from build123d import *

# Parameters (mm, degrees)
SKETCH1_W           = 50.8
SKETCH1_H           = 50.8
SKETCH1_W_2         = 44.45
BOSS_EXTRUDE1_DEPTH = 6.35
FILLET2_R           = 3.175
SKETCH2_R           = 6.35
BOSS_EXTRUDE3_DEPTH = 6.35
BOSS_EXTRUDE4_START = -6.35
SKETCH4_R           = 6.35
BOSS_EXTRUDE4_DEPTH = 6.35
CUT_EXTRUDE1_REACH  = 164.453
SKETCH2_4_R         = 4.49961
SKETCH2_4_R_2       = 1.9939
BOSS_EXTRUDE5_DEPTH = 127


with BuildPart() as part:
    # Sketch1 → Boss-Extrude1 (new body)
    with BuildSketch(Plane(origin=(0, 0, 0), x_dir=(1, 0, 0), z_dir=(0, 1, 0))):
        Polygon((-146.05, 25.4), (-127, 25.4), (-127, -25.4), (-146.05, -25.4), (-146.05, -31.75), (146.05, -31.75), (146.05, -25.4), (127, -25.4), (127, 25.4), (146.05, 25.4), (146.05, 31.75), (-146.05, 31.75), align=None)
        with Locations((-31.75, 0)):
            Rectangle(SKETCH1_W, SKETCH1_H, mode=Mode.SUBTRACT)
        with Locations((-92.075, 0)):
            Rectangle(SKETCH1_W_2, SKETCH1_H, mode=Mode.SUBTRACT)
        with Locations((31.75, 0)):
            Rectangle(SKETCH1_W, SKETCH1_H, mode=Mode.SUBTRACT)
        with Locations((92.075, 0)):
            Rectangle(SKETCH1_W_2, SKETCH1_H, mode=Mode.SUBTRACT)
    extrude(amount=-BOSS_EXTRUDE1_DEPTH)

    # Fillet2
    fillet2_edges = [part.edges().sort_by_distance(p)[0] for p in [
        (-146.05, -6.35, 28.575),
        (-146.05, 0, 28.575),
        (-146.05, -6.35, -28.575),
        (-146.05, 0, -28.575),
        (146.05, -6.35, -28.575),
        (146.05, 0, -28.575),
        (146.05, -6.35, 28.575),
        (146.05, 0, 28.575),
    ]]
    fillet(fillet2_edges, radius=FILLET2_R - 0.0001)  # a hair under: the kernel refuses the full size

    # Sketch2 → Boss-Extrude3 (add)
    with BuildSketch(Plane.XY.offset(31.75)):
        with Locations((-142.875, -3.175)):
            Circle(SKETCH2_R)
    extrude(amount=-BOSS_EXTRUDE3_DEPTH)

    # Sketch4 → Boss-Extrude4 (add)
    with BuildSketch(Plane(origin=(0, 0, -31.75), x_dir=(-1, 0, 0), z_dir=(0, 0, -1)).offset(BOSS_EXTRUDE4_START)):
        with Locations((142.875, -3.175)):
            Circle(SKETCH4_R)
    extrude(amount=BOSS_EXTRUDE4_DEPTH)

    # Cut-Extrude1: up to this face of the body (flat: up to its plane)
    cut_extrude1_end = Plane(part.part.faces().sort_by_distance((-5.43222234, -3.175, -31.75))[0])
    # Sketch2<4> → Cut-Extrude1 (cut, up to the picked face)
    with BuildSketch(Plane.XY.offset(31.75), mode=Mode.PRIVATE) as cut_extrude1_sk1:
        with Locations((-142.875, -3.175)):
            Circle(SKETCH2_4_R)
    cut_extrude1_tool1 = split(extrude(cut_extrude1_sk1.sketch, amount=-CUT_EXTRUDE1_REACH, mode=Mode.PRIVATE), bisect_by=cut_extrude1_end, keep=Keep.BOTH, mode=Mode.PRIVATE)
    # Sketch2<4> → Cut-Extrude1 (cut, up to the picked face)
    with BuildSketch(Plane.XY.offset(31.75), mode=Mode.PRIVATE) as cut_extrude1_sk2:
        with Locations((-92.075, -3.175)):
            Circle(SKETCH2_4_R_2)
    cut_extrude1_tool2 = split(extrude(cut_extrude1_sk2.sketch, amount=-CUT_EXTRUDE1_REACH, mode=Mode.PRIVATE), bisect_by=cut_extrude1_end, keep=Keep.BOTH, mode=Mode.PRIVATE)
    # Sketch2<4> → Cut-Extrude1 (cut, up to the picked face)
    with BuildSketch(Plane.XY.offset(31.75), mode=Mode.PRIVATE) as cut_extrude1_sk3:
        with Locations((-31.75, -3.175)):
            Circle(SKETCH2_4_R_2)
    cut_extrude1_tool3 = split(extrude(cut_extrude1_sk3.sketch, amount=-CUT_EXTRUDE1_REACH, mode=Mode.PRIVATE), bisect_by=cut_extrude1_end, keep=Keep.BOTH, mode=Mode.PRIVATE)
    # Sketch2<4> → Cut-Extrude1 (cut, up to the picked face)
    with BuildSketch(Plane.XY.offset(31.75), mode=Mode.PRIVATE) as cut_extrude1_sk4:
        with Locations((31.75, -3.175)):
            Circle(SKETCH2_4_R_2)
    cut_extrude1_tool4 = split(extrude(cut_extrude1_sk4.sketch, amount=-CUT_EXTRUDE1_REACH, mode=Mode.PRIVATE), bisect_by=cut_extrude1_end, keep=Keep.BOTH, mode=Mode.PRIVATE)
    # Sketch2<4> → Cut-Extrude1 (cut, up to the picked face)
    with BuildSketch(Plane.XY.offset(31.75), mode=Mode.PRIVATE) as cut_extrude1_sk5:
        with Locations((92.075, -3.175)):
            Circle(SKETCH2_4_R_2)
    cut_extrude1_tool5 = split(extrude(cut_extrude1_sk5.sketch, amount=-CUT_EXTRUDE1_REACH, mode=Mode.PRIVATE), bisect_by=cut_extrude1_end, keep=Keep.BOTH, mode=Mode.PRIVATE)
    # Sketch2<4> → Cut-Extrude1 (cut, up to the picked face)
    with BuildSketch(Plane.XY.offset(31.75), mode=Mode.PRIVATE) as cut_extrude1_sk6:
        with Locations((-120.65, -3.175)):
            Circle(SKETCH2_4_R_2)
    cut_extrude1_tool6 = split(extrude(cut_extrude1_sk6.sketch, amount=-CUT_EXTRUDE1_REACH, mode=Mode.PRIVATE), bisect_by=cut_extrude1_end, keep=Keep.BOTH, mode=Mode.PRIVATE)
    # Sketch2<4> → Cut-Extrude1 (cut, up to the picked face)
    with BuildSketch(Plane.XY.offset(31.75), mode=Mode.PRIVATE) as cut_extrude1_sk7:
        with Locations((61.9125, -3.175)):
            Circle(SKETCH2_4_R_2)
    cut_extrude1_tool7 = split(extrude(cut_extrude1_sk7.sketch, amount=-CUT_EXTRUDE1_REACH, mode=Mode.PRIVATE), bisect_by=cut_extrude1_end, keep=Keep.BOTH, mode=Mode.PRIVATE)
    # Sketch2<4> → Cut-Extrude1 (cut, up to the picked face)
    with BuildSketch(Plane.XY.offset(31.75), mode=Mode.PRIVATE) as cut_extrude1_sk8:
        with BuildLine():
            Line((135.255, -1.1811), (142.875, -1.1811))
            ThreePointArc((142.875, -1.1811), (144.8689, -3.175), (142.875, -5.1689))
            Line((142.875, -5.1689), (135.255, -5.1689))
            ThreePointArc((135.255, -5.1689), (133.2611, -3.175), (135.255, -1.1811))
        make_face()
    cut_extrude1_tool8 = split(extrude(cut_extrude1_sk8.sketch, amount=-CUT_EXTRUDE1_REACH, mode=Mode.PRIVATE), bisect_by=cut_extrude1_end, keep=Keep.BOTH, mode=Mode.PRIVATE)
    add(cut_extrude1_tool1.solids().sort_by(Axis((-142.875, -3.175, 31.75), (0, 0, -1)))[0], mode=Mode.SUBTRACT)
    add(cut_extrude1_tool2.solids().sort_by(Axis((-92.075, -3.175, 31.75), (0, 0, -1)))[0], mode=Mode.SUBTRACT)
    add(cut_extrude1_tool3.solids().sort_by(Axis((-31.75, -3.175, 31.75), (0, 0, -1)))[0], mode=Mode.SUBTRACT)
    add(cut_extrude1_tool4.solids().sort_by(Axis((31.75, -3.175, 31.75), (0, 0, -1)))[0], mode=Mode.SUBTRACT)
    add(cut_extrude1_tool5.solids().sort_by(Axis((92.075, -3.175, 31.75), (0, 0, -1)))[0], mode=Mode.SUBTRACT)
    add(cut_extrude1_tool6.solids().sort_by(Axis((-120.65, -3.175, 31.75), (0, 0, -1)))[0], mode=Mode.SUBTRACT)
    add(cut_extrude1_tool7.solids().sort_by(Axis((61.9125, -3.175, 31.75), (0, 0, -1)))[0], mode=Mode.SUBTRACT)
    add(cut_extrude1_tool8.solids().sort_by(Axis((139.065, -3.175, 31.75), (0, 0, -1)))[0], mode=Mode.SUBTRACT)

    # Sketch5 → Boss-Extrude5 (add)
    with BuildSketch(Plane(origin=(127, 0, 0), x_dir=(0, 0, -1), z_dir=(1, 0, 0))):
        Polygon((25.4, -6.35), (31.75, -6.35), (28.575, -9.525), align=None)
        Polygon((-31.75, -6.35), (-25.4, -6.35), (-28.575, -9.525), align=None)
    extrude(amount=-BOSS_EXTRUDE5_DEPTH)


solid = part.part
The model under review builds one solid part; all positions refer to its coordinate system, in mm. A direction names the side the tool comes from. Coordinates: 2 decimals unless noted, no trailing zeros. Order: outer loops, then holes, each group sorted by start corner. A loop starts at its lowest first (then second) coordinate and runs counter-clockwise, first axis right, second up. Notation, with made-up numbers: (-40, -22.75) -> (-32, -22.75) arc R29 ccw to (-32, 12.25) -> close; hole circle Ø5 at (47, -34). An arc over 180 degrees is marked (long way). Answer in a Markdown table with one row per item.
(1) Consider section B-B (x = 21). Write out the cut boundary in (y, z) (3 decimals), plus the area to 3 significant figures.
Answers:
| item | result |
|---|---|
| outline | (-9.525, -28.575) -> (-6.35, -31.75) -> (0, -31.75) -> (0, -25.4) -> (-6.35, -25.4) -> close; (-9.525, 28.575) -> (-6.35, 25.4) -> (0, 25.4) -> (0, 31.75) -> (-6.35, 31.75) -> close |
| area | 101 mm² |
(2) Insertion check: pin 1 (1.9 mm diameter, centred on y = -1.5, z = -0.5, fed in from +X); pin 2 (5 mm diameter, centred on y = -4.5, z = -12.5, fed in from -X); pin 3 (1.9 mm diameter, centred on x = 139.5, z = 28.5, fed in from +Y); pin 4 (6.5 mm diameter, centred on x = 92.075, y = -3.175, fed in from -Z). Each pin has a flat end and moves straight along its axis. Give the tip position at first contact, or say it passes through.
Answers:
| item | result |
|---|---|
| pin 1 | x = 127 |
| pin 2 | x = -127 |
| pin 3 | y = 0 |
| pin 4 | z = -31.75 |
(3) Machinability: for faces 4 (the flat face through (63, -6.35, 0)), 5 (the flat face through (-138, -3, 25.4)), 6 (the flat face through (135, -6.35, -29)), which of the approach directions +Z, -Z, +X, -X, +Y, -Y give a long, thin tool a straight path to every point of the face, cutting with its end or side? Answer none if there is none.
Answers:
| item | result |
|---|---|
| face 4 | +X, -X, -Y |
| face 5 | -X, +Y, -Y |
| face 6 | +Z, -Z, +X, -Y |
(4) Consider section A-A (z = -4). State how many separate pieces and enclosed holes the cut face has, plus the area to 3 significant figures.
Answers:
| item | result |
|---|---|
| separate pieces | 5 |
| enclosed holes | 2 |
| area | 378 mm² |
(5) Wall thickness on line 1 along X through (y, z) = (-1, 18.5); line 2 along Z through (x, y) = (-11.5, -1); line 3 along Y through (x, z) = (-120.65, -10.5): over which ranges is each line inside the solid? List them lowest first.
Answers:
| item | result |
|---|---|
| line 1 | -127 to -114.3, -69.85 to -57.15, -6.35 to 6.35, 57.15 to 69.85, 114.3 to 127 |
| line 2 | -31.75 to -25.4, 25.4 to 31.75 |
| line 3 | -6.35 to -5.17, -1.18 to 0 |
(6) The part is to be moulded in two halves that separate along X. For faces 1 (the flat face through (135, -6.35, 29)), 2 (the flat face through (92, -1, 25.4)), 3 (the flat face through (-127, -3, 0)), say which applies: +X half, -X half, draft (parallel to the pull), parting line (faces both ways), or undercut.
Answers:
| item | result |
|---|---|
| face 1 | draft |
| face 2 | undercut |
| face 3 | -X half |
